Check sheet for the drawn part. Datum: minimum x, y, z corner. Units: mm. Give positions to 0.01 mm unless a question says otherwise; leave off trailing zeros. Write each loop counter-clockwise with the first axis right and the second up, starting at its lowest first coordinate (ties: lowest second). Pieces come first, ordered by that corner, then holes. Notation, with made-up numbers: M 11.25,47 L 47.25,47 A16 ccw 47.25,59 Z; hole C 30.5,32 d4. An arc over 180 degrees is marked long. Write item = value, one per line.
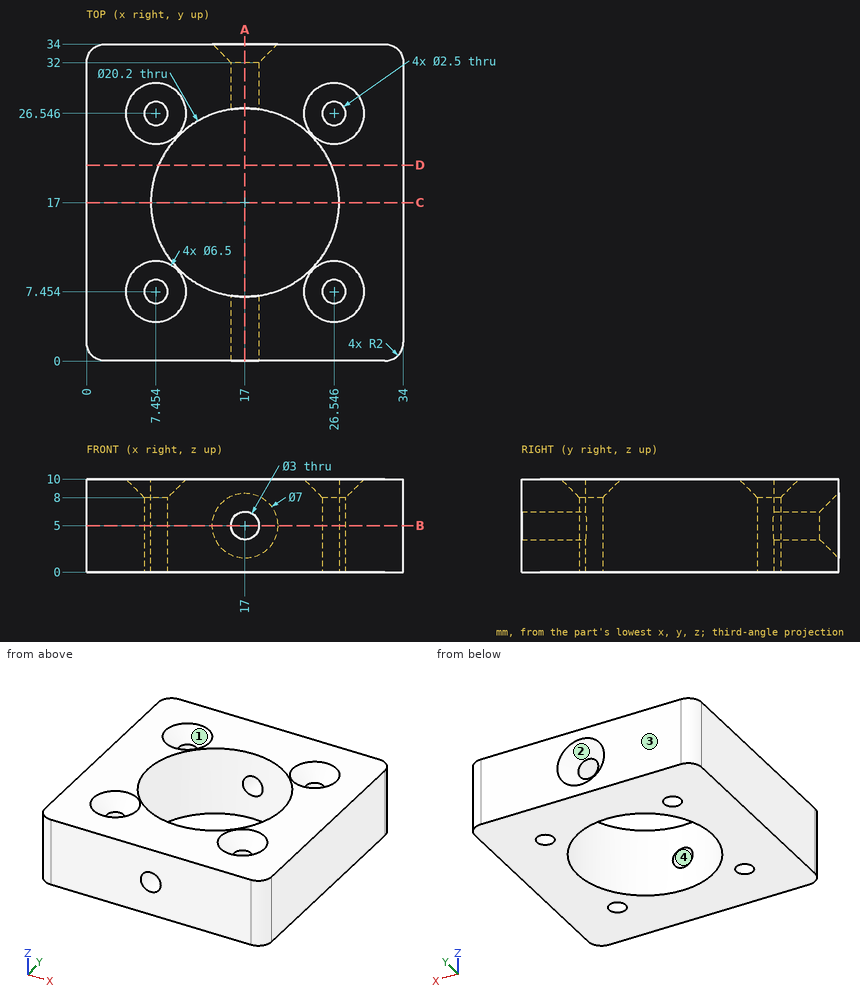
1) Cross-section at A-A on x = 17. Record the boundary of the cut face in (y, z), plus the area to 3 significant figures.
From the geometry:
outline = M 0,0 L 6.9,0 L 6.9,3.5 L 0,3.5 Z; M 0,6.5 L 6.9,6.5 L 6.9,10 L 0,10 Z; M 27.1,0 L 34,0 L 34,1.5 L 32,3.5 L 27.1,3.5 Z; M 27.1,6.5 L 32,6.5 L 34,8.5 L 34,10 L 27.1,10 Z
area = 92.6 mm^2
2) Cross-section at D-D on y = 21. Record the boundary of the cut face in (x, z).
From the geometry:
outline = M 0,0 L 7.73,0 L 7.73,10 L 0,10 Z; M 26.27,0 L 34,0 L 34,10 L 26.27,10 Z
3) Depth check by flat-ended pin: P1, Ø4, axis at x = 7.45, y = 7.45, coming from the +Z side; P2, Ø4, axis at x = 7.45, y = 26.55, coming from the -Z side; P3, Ø3, axis at x = 26.55, y = 26.55, coming from the +Z side. Enter the tip coordinate at first touch or a pass-through.
From the geometry:
P1 = 8.76
P2 = 0
P3 = 8.26
4) Cross-section at C-C on y = 17. Record the boundary of the cut face in (x, z), plus the area to 3 significant figures.
From the geometry:
outline = M 0,0 L 6.9,0 L 6.9,10 L 0,10 Z; M 27.1,0 L 34,0 L 34,10 L 27.1,10 Z
area = 138 mm^2
5) Cross-section at B-B on z = 5. Record the boundary of the cut face in (x, y), plus the area to 3 significant figures.
From the geometry:
outline = M 0,2 A2 ccw 2,0 L 15.5,0 L 15.5,7.01 A10.1 cw 15.5,26.99 L 15.5,32 L 13.5,34 L 2,34 A2 ccw 0,32 Z; M 18.5,0 L 32,0 A2 ccw 34,2 L 34,32 A2 ccw 32,34 L 20.5,34 L 18.5,32 L 18.5,26.99 A10.1 cw 18.5,7.01 Z; hole C 7.45,7.45 d2.5; hole C 7.45,26.55 d2.5; hole C 26.55,7.45 d2.5; hole C 26.55,26.55 d2.5
area = 767 mm^2
6) Material ranges on probe 1 along Y at (x, z) = (27.5, 5); probe 2 along Y at (x, z) = (16.5, 3.5), recorded low to high. Write a range as from..to.
From the geometry:
probe_1 = 0..6.65, 8.26..25.74, 27.35..34
probe_2 = 0..6.91, 27.09..32.08
7) Draft check along Z on the marked faces 1, 2, 3 and 4. Enter one of: +Z half, -Z half, draft (parallel to the pull), parting line (faces both ways), or undercut.
From the geometry:
face_1 = +Z half
face_2 = undercut
face_3 = draft
face_4 = undercut
